For this review, take the finished solid that the model builds, in its own axes (mm). Face numbers are marked on the shaded views. A direction names the side the tool comes from. Round coordinates to 2 decimals unless told otherwise and drop trailing zeros. Loops run counter-clockwise (first coordinate to the right, second up) from the corner with the lowest first, then second, coordinate; pieces in that order, holes last.
1) Wall thickness on L1, parallel to X at y = 2.25, z = 1; L2, parallel to Z at x = -1.25, y = 0; L3, parallel to X at y = -3.5, z = -1.5: over which ranges is each line inside the solid? List them lowest first.
2) Take a section at D-D (x = -16.25). State the section outline as (y, z) points.
3) Insertion check: pin 1 (1 mm diameter, centred on x = -18.5, z = 2, fed in from +Y); pin 2 (1.5 mm diameter, centred on x = -19.5, y = 0, fed in from -Z); pin 3 (1.5 mm diameter, centred on x = -27.5, z = 0.5, fed in from -Y). Each pin has a flat end and moves straight along its axis. Give the tip position at first contact, or say it passes through.
4) Take a section at A-A (y = 0). State the section outline as (x, z) points.
5) Mouldability with a two-part tool opening along Y and no side actions: class the marked faces 5, 6 and 7 as pulls with the +Y half, pulls with the -Y half, needs draft (parallel to the pull), parting line crosses it, or undercut.
6) Tool access review of the marked faces 1, 2, 3 and 4: name each direction out of +Z, -Z, +X, -X, +Y, -Y from which nothing blocks a thin tool from reaching the whole face with its end or side.
7) Take a section at B-B (z = 0). State the section outline as (x, y) points.
8) Take a section at C-C (x = -23.5). State the section outline as (y, z) points.
```python
from build123d import *

# Parameters (mm, degrees)
F0_R      = 5.334
F1_DEPTH  = 6.4262
F2_R      = 3.9624
F3_DEPTH  = 13.3858
F5_DEPTH  = 5.588
F7_DEPTH  = 3.048
F8_SIZE2  = 0.762
F8_SIZE   = 0.762
F9_R      = 2.38125
F10_DEPTH = 7.874
F13_D     = 2.2606
F13_DEPTH = 6.477
F13_START = 0.1211335
F13_TIP   = 0.6791527577
F16_D     = 2.2606
F16_DEPTH = 6.477
F16_START = 0.1211335
F16_TIP   = 0.6791527577


with BuildPart() as f1:
    # F0 (on Right) → F1 (new body)
    with BuildSketch(Plane.YZ):
        Circle(F0_R)
    extrude(amount=-F1_DEPTH)

    # F2 (on face) → F3 (join)
    with BuildSketch(Plane(origin=(-6.4262, 0, 0), x_dir=(0, -1, 0), z_dir=(-1, 0, 0))):
        Circle(F2_R)
    extrude(amount=F3_DEPTH)

    # F4 (on face) → F5 (join)
    with BuildSketch(Plane(origin=(-19.812, 0, 0), x_dir=(0, -1, 0), z_dir=(-1, 0, 0))):
        with BuildLine():
            Line((3.4148820894, 1.6895799227), (-1.4267371035, 3.5327781189))
            ThreePointArc((-1.4267371035, 3.5327781189), (-1.5592731706, 3.4763151726), (-1.6895799227, 3.4148820894))
            Line((-1.6895799227, 3.4148820894), (-3.5327781189, -1.4267371035))
            ThreePointArc((-3.5327781189, -1.4267371035), (-3.4763151726, -1.5592731706), (-3.4148820894, -1.6895799227))
            Line((-3.4148820894, -1.6895799227), (1.4267371035, -3.5327781189))
            ThreePointArc((1.4267371035, -3.5327781189), (1.5592731706, -3.4763151726), (1.6895799227, -3.4148820894))
            Line((1.6895799227, -3.4148820894), (3.5327781189, 1.4267371035))
            ThreePointArc((3.5327781189, 1.4267371035), (3.4763151726, 1.5592731706), (3.4148820894, 1.6895799227))
        make_face()
    extrude(amount=F5_DEPTH)

    # F6 (on face) → F7 (join)
    with BuildSketch(Plane(origin=(-25.4, 0, 0), x_dir=(0, -1, 0), z_dir=(-1, 0, 0))):
        with BuildLine():
            Line((1.5748, -1.7606799255), (1.5748, 1.7606799255))
            ThreePointArc((1.5748, 1.7606799255), (-2.3622, 0), (1.5748, -1.7606799255))
        make_face()
    extrude(amount=F7_DEPTH)

    # F8
    f8_edges = [f1.edges().sort_by_distance(p)[0] for p in [
        (0, -5.334, 0),
    ]]
    chamfer(f8_edges, length=F8_SIZE, length2=F8_SIZE2)

    # F9 (on face) → F10 (cut)
    with BuildSketch(Plane.YZ):
        Circle(F9_R)
    extrude(amount=-F10_DEPTH, mode=Mode.SUBTRACT)

    # F13
    # its depths count from where the whole tool has entered the part; down to there all is cleared
    with Locations(Plane.XZ.offset(5.334).offset(-F13_START)):
        with Locations((-3.3782, 0)):
            Hole(F13_D / 2, depth=F13_DEPTH)
            with Locations((0, 0, -(F13_DEPTH + F13_TIP / 2))):  # 118° drill point
                Cone(0, F13_D / 2, F13_TIP, mode=Mode.SUBTRACT)

    # F16
    # its depths count from where the whole tool has entered the part; down to there all is cleared
    with Locations(Plane.XY.offset(5.334).offset(-F16_START)):
        with Locations((-3.3782, 0)):
            Hole(F16_D / 2, depth=F16_DEPTH)
            with Locations((0, 0, -(F16_DEPTH + F16_TIP / 2))):  # 118° drill point
                Cone(0, F16_D / 2, F16_TIP, mode=Mode.SUBTRACT)


solid = f1.part
```
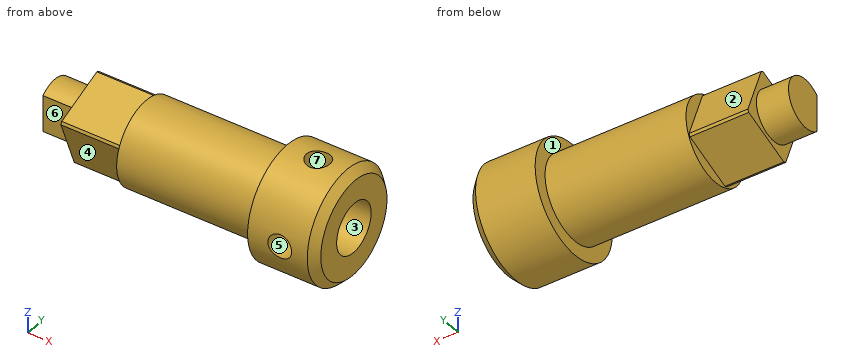
Response:
1. L1: x = -25.4 to 0
1. L2: z = -5.33 to -2.38, 2.38 to 5.33
1. L3: x = -19.81 to 0
2. outline: circle Ø7.92 at (0, 0)
3. pin 1: stops at y = 3.67
3. pin 2: stops at z = -3.96
3. pin 3: stops at y = -1.57
4. outline: (-28.45, -2.36) - (-25.4, -2.36) - (-25.4, -2.99) - (-19.81, -2.99) - (-19.81, -3.96) - (-6.43, -3.96) - (-6.43, -5.33) - (-0.76, -5.33) - (0, -4.57) - (0, -2.38) - (-7.87, -2.38) - (-7.87, 2.38) - (-4.51, 2.38) - (-4.51, 5.33) - (-6.43, 5.33) - (-6.43, 3.96) - (-19.81, 3.96) - (-19.81, 2.99) - (-25.4, 2.99) - (-25.4, 2.36) - (-28.45, 2.36) - close; (-2.25, 2.38) - (0, 2.38) - (0, 4.57) - (-0.76, 5.33) - (-2.25, 5.33) - close
5. face 5: needs draft
5. face 6: pulls with the -Y half
5. face 7: undercut
6. face 1: -X
6. face 2: +Z, -X, +Y
6. face 3: +X
6. face 4: -Z, -X, -Y
7. outline: (-28.45, -1.57) - (-25.4, -1.57) - (-25.4, -2.99) - (-19.81, -2.99) - (-19.81, -3.96) - (-6.43, -3.96) - (-6.43, -5.33) - (-4.51, -5.33) - (-4.51, -2.38) - (-7.87, -2.38) - (-7.87, 2.38) - (0, 2.38) - (0, 4.57) - (-0.76, 5.33) - (-6.43, 5.33) - (-6.43, 3.96) - (-19.81, 3.96) - (-19.81, 2.99) - (-25.4, 2.99) - (-25.4, 2.36) - (-28.45, 2.36) - close; (-2.25, -5.33) - (-0.76, -5.33) - (0, -4.57) - (0, -2.38) - (-2.25, -2.38) - close
8. outline: (-3.53, 1.43) - (-1.69, -3.41) arc R3.81 ccw to (-1.43, -3.53) - (3.41, -1.69) arc R3.81 ccw to (3.53, -1.43) - (1.69, 3.41) arc R3.81 ccw to (1.43, 3.53) - (-3.41, 1.69) arc R3.81 ccw to start
